Design review of the part built by this model. Coordinates are the model's own, in mm. Round coordinates to 2 decimals unless told otherwise and drop trailing zeros. Write item = value, one per line.
from build123d import *

# Parameters (mm, degrees)
SKETCH1_W           = 100
SKETCH1_H           = 100
BOSS_EXTRUDE1_DEPTH = 50
CHAMFER1_SIZE       = 3
SKETCH3_W           = 100
SKETCH3_H           = 1.369103339
CUT_EXTRUDE1_DEPTH  = 25
SKETCH4_W           = 72
SKETCH4_H           = 1.369103339
SKETCH4_W_2         = 3
SKETCH4_W_3         = 75
CUT_EXTRUDE2_DEPTH  = 25
SKETCH5_W           = 75
SKETCH5_H           = 1.369103339
CUT_EXTRUDE3_DEPTH  = 25


with BuildPart() as part:
    # Sketch1 → Boss-Extrude1 (new body)
    with BuildSketch(Plane(origin=(0, 0, 0), x_dir=(1, 0, 0), z_dir=(0, 1, 0))):
        with Locations((50, -50)):
            Rectangle(SKETCH1_W, SKETCH1_H)
    extrude(amount=BOSS_EXTRUDE1_DEPTH)

    # Chamfer1
    chamfer1_edges = [part.edges().sort_by_distance(p)[0] for p in [
        (0, 25, 0),
        (100, 25, 0),
        (100, 25, 100),
        (0, 25, 100),
    ]]
    chamfer(chamfer1_edges, length=CHAMFER1_SIZE)

    # Sketch3 → Cut-Extrude1 (cut)
    with BuildSketch(Plane.ZY):
        with Locations((50, 43.425849107)):
            Rectangle(SKETCH3_W, SKETCH3_H)
        with Locations((50, 37.425849107)):
            Rectangle(SKETCH3_W, SKETCH3_H)
        with Locations((50, 31.425849107)):
            Rectangle(SKETCH3_W, SKETCH3_H)
        with Locations((50, 25.425849107)):
            Rectangle(SKETCH3_W, SKETCH3_H)
        with Locations((50, 19.425849107)):
            Rectangle(SKETCH3_W, SKETCH3_H)
        with Locations((50, 13.425849107)):
            Rectangle(SKETCH3_W, SKETCH3_H)
        with Locations((50, 7.425849108)):
            Rectangle(SKETCH3_W, SKETCH3_H)
    extrude(amount=-CUT_EXTRUDE1_DEPTH, mode=Mode.SUBTRACT)

    # Sketch4 → Cut-Extrude2 (cut)
    with BuildSketch(Plane.XY.offset(100)):
        with Locations((61, 25.425849107)):
            Rectangle(SKETCH4_W, SKETCH4_H)
        with Locations((61, 19.425849107)):
            Rectangle(SKETCH4_W, SKETCH4_H)
        with Locations((61, 13.425849107)):
            Rectangle(SKETCH4_W, SKETCH4_H)
        with Locations((98.5, 25.425849107)):
            Rectangle(SKETCH4_W_2, SKETCH4_H)
        with Locations((98.5, 19.425849107)):
            Rectangle(SKETCH4_W_2, SKETCH4_H)
        with Locations((98.5, 13.425849107)):
            Rectangle(SKETCH4_W_2, SKETCH4_H)
        with Locations((62.5, 7.425849108)):
            Rectangle(SKETCH4_W_3, SKETCH4_H)
        with Locations((62.5, 31.425849107)):
            Rectangle(SKETCH4_W_3, SKETCH4_H)
        with Locations((62.5, 37.425849107)):
            Rectangle(SKETCH4_W_3, SKETCH4_H)
        with Locations((62.5, 43.425849107)):
            Rectangle(SKETCH4_W_3, SKETCH4_H)
    extrude(amount=-CUT_EXTRUDE2_DEPTH, mode=Mode.SUBTRACT)

    # Sketch5 → Cut-Extrude3 (cut)
    with BuildSketch(Plane(origin=(0, 0, 0), x_dir=(-1, 0, 0), z_dir=(0, 0, -1))):
        with Locations((-62.5, 43.425849107)):
            Rectangle(SKETCH5_W, SKETCH5_H)
        with Locations((-62.5, 37.425849107)):
            Rectangle(SKETCH5_W, SKETCH5_H)
        with Locations((-62.5, 31.425849107)):
            Rectangle(SKETCH5_W, SKETCH5_H)
        with Locations((-62.5, 25.425849107)):
            Rectangle(SKETCH5_W, SKETCH5_H)
        with Locations((-62.5, 19.425849107)):
            Rectangle(SKETCH5_W, SKETCH5_H)
        with Locations((-62.5, 13.425849107)):
            Rectangle(SKETCH5_W, SKETCH5_H)
        with Locations((-62.5, 7.425849108)):
            Rectangle(SKETCH5_W, SKETCH5_H)
    extrude(amount=-CUT_EXTRUDE3_DEPTH, mode=Mode.SUBTRACT)


solid = part.part
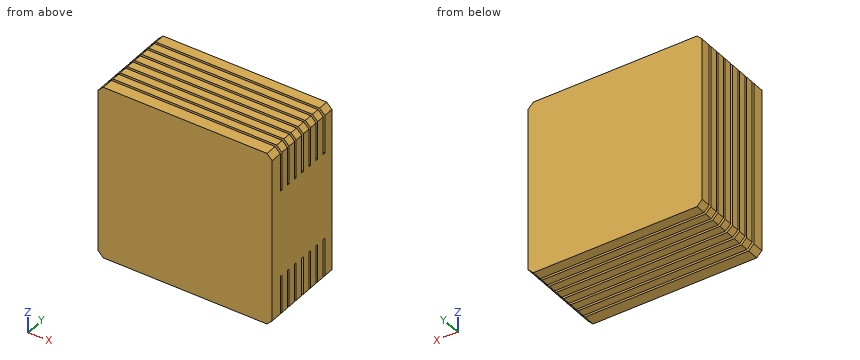
Item 1: For line 1 along Z through (x, y) = (82.5, 20); line 2 along X through (y, z) = (7, 63.5), list the stretches that pass through material, from the lowest coordinate up. Write a range as [from, to].
Data:
line_1 = [25, 75]
line_2 = [25, 100]
Item 2: Take a section at A-A, the plane x = 17. Count the separate pieces of the cut face and the enclosed holes in it, and give its area (3 significant figures).
Data:
separate_pieces = 8
enclosed_holes = 0
area = 4,040 mm2
Item 3: Insertion check: P1, Ø1.1, axis at x = 64.5, y = 7.5, coming from the -Z side; P2, Ø5, axis at y = 42, z = 54.5, coming from the -X side; P3, Ø0.7, axis at y = 37.5, z = 57.5, coming from the -X side. Each pin has a flat end and moves straight along its axis. Give the tip position at first contact, or say it passes through.
Data:
P1 = 25
P2 = 0
P3 = 25
